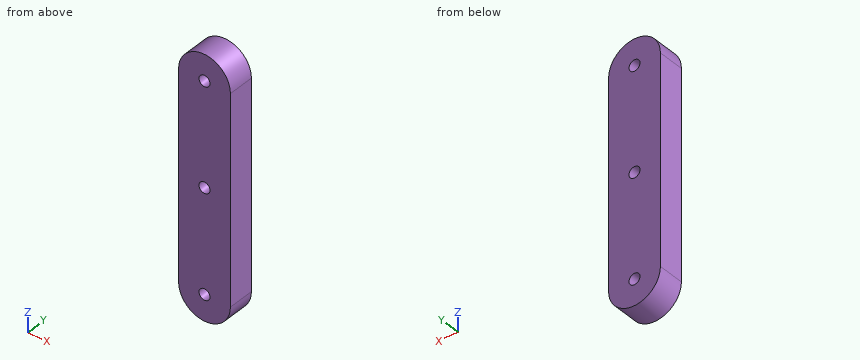
from build123d import *

# Parameters (mm, degrees)
BOSS_EXTRUDE1_DEPTH   = 6.35
F_6_32_TAPPED_HOLE1_D = 2.7051


with BuildPart() as part:
    # Sketch1 → Boss-Extrude1 (new body)
    with BuildSketch(Plane(origin=(0, 0, 0), x_dir=(1, 0, 0), z_dir=(0, 1, 0))):
        with BuildLine():
            Line((-6.35, -25.4), (-6.35, 25.4))
            ThreePointArc((-6.35, 25.4), (0, 31.75), (6.35, 25.4))
            Line((6.35, 25.4), (6.35, -25.4))
            ThreePointArc((6.35, -25.4), (0, -31.75), (-6.35, -25.4))
        make_face()
    extrude(amount=BOSS_EXTRUDE1_DEPTH)

    # #6-32 Tapped Hole1 (through all)
    with Locations(Plane(origin=(0, 6.35, 0), x_dir=(1, 0, 0), z_dir=(0, 1, 0))):
        with Locations((0, -25.4), (0, 25.4), (0, 0)):
            Hole(F_6_32_TAPPED_HOLE1_D / 2)


solid = part.part
Read the model definition and answer for the solid it produces. Units are mm, in the model's axes. Give positions to 0.01 mm unless a question says otherwise; leave off trailing zeros. Write each loop counter-clockwise with the first axis right and the second up, starting at its lowest first coordinate (ties: lowest second). Pieces come first, ordered by that corner, then holes. Notation, with made-up numbers: (35.25, -30.5) -> (73.25, -30.5) arc R30 cw to (73.25, -1.5) -> close; hole circle Ø8 at (2, -15). An arc over 180 degrees is marked (long way). Answer as a JSON object with one key per item and string values. Group by question number.
1) Find section D-D (x = 3). Write down the section's boundary in (y, z), and give its area (3 significant figures).
2) Consider L1, parallel to Z at x = 0, y = 3; L2, parallel to Z at x = 1, y = 2; L3, parallel to X at y = 1.5, z = -25.4. Determine where each line is inside the solid, lowest interval first. Write a range as from..to.
3) Each of these flat-tipped pins is pushed along its axis until it touches: P1, Ø3, axis at x = 3.5, y = 3.5, coming from the -Z side; P2, Ø3, axis at x = -2.5, y = 4, coming from the +Z side; P3, Ø2, axis at x = 0, z = 0, coming from the +Y side. Where does it stop, or does it pass through?
4) Find section C-C (x = 0). Write down the section's boundary in (y, z), and give its area (3 significant figures).
5) Find section A-A (z = 0). Write down the section's boundary in (x, y).
6) Find section B-B (y = 4.75). Write down the section's boundary in (x, z).
Values follow:
{
 "1": {"outline": "(0, -31) -> (6.35, -31) -> (6.35, 31) -> (0, 31) -> close", "area": "394 mm2"},
 "2": {"L1": "z = -31.75..-26.75, -24.05..-1.35, 1.35..24.05, 26.75..31.75", "L2": "z = -31.67..-26.31, -24.49..-0.91, 0.91..24.49, 26.31..31.67", "L3": "x = -6.35..-1.35, 1.35..6.35"},
 "3": {"P1": "stops at z = -31.43", "P2": "stops at z = 31.67", "P3": "passes through"},
 "4": {"outline": "(0, -31.75) -> (6.35, -31.75) -> (6.35, -26.75) -> (0, -26.75) -> close; (0, -24.05) -> (6.35, -24.05) -> (6.35, -1.35) -> (0, -1.35) -> close; (0, 1.35) -> (6.35, 1.35) -> (6.35, 24.05) -> (0, 24.05) -> close; (0, 26.75) -> (6.35, 26.75) -> (6.35, 31.75) -> (0, 31.75) -> close", "area": "352 mm2"},
 "5": {"outline": "(-6.35, 0) -> (-1.35, 0) -> (-1.35, 6.35) -> (-6.35, 6.35) -> close; (1.35, 0) -> (6.35, 0) -> (6.35, 6.35) -> (1.35, 6.35) -> close"},
 "6": {"outline": "(-6.35, -25.4) arc R6.35 ccw to (6.35, -25.4) -> (6.35, 25.4) arc R6.35 ccw to (-6.35, 25.4) -> close; hole circle Ø2.71 at (0, -25.4); hole circle Ø2.71 at (0, 0); hole circle Ø2.71 at (0, 25.4)"}
}
